Read the model definition and answer for the solid it produces. Units are mm, in the model's axes. A direction names the side the tool comes from. Give positions to 0.01 mm unless a question says otherwise; leave off trailing zeros. Write each loop counter-clockwise with the first axis right and the second up, starting at its lowest first coordinate (ties: lowest second). Pieces come first, ordered by that corner, then holes. Notation, with made-up numbers: M 42,26 L 49,26 A36 cw 49,62 Z; hole C 57.25,-10.75 d8. An arc over 180 degrees is marked long. Use a Markdown table: item, result. Add a question column.
Item 1: A cutting plane is placed at B-B on y = 1. Determine the outline of the cut face in (x, z), then the cut area to 3 significant figures.
Item 2: A cutting plane is placed at D-D on z = 2.25. Determine the outline of the cut face in (x, y).
Item 3: A cutting plane is placed at A-A on z = 4.25. Determine the outline of the cut face in (x, y), then the cut area to 3 significant figures.
Item 4: Consider probe 1 along X at (y, z) = (4.5, -2.25); probe 2 along X at (y, z) = (5.25, 3.5); probe 3 along X at (y, z) = (8.5, -5.25). Determine where each line is inside the solid, lowest interval first. Write a range as [from, to].
Item 5: A cutting plane is placed at C-C on y = 7.5. Determine the outline of the cut face in (x, z), then the cut area to 3 significant figures.
Item 6: For faces 1 (the flat face through (4, 15, 0)), 2 (the flat face through (-8, 8, -3.027)), determine the directions among +Z, -Z, +X, -X, +Y, -Y from which every point of the face is accessible in a straight line to the end or side of a thin tool.
Item 7: The mould has two halves that part along X. Classify faces 3 (the flat face through (17.5, 7, 0)), 4 (the cylindrical face through (-15.273, 7.906, 5.479)), 5 (the flat face through (-8, 6, 3.027)), 6 (the cylindrical face through (-11.704, 8.852, 5.548)): pulls with the +X half, pulls with the -X half, needs draft (parallel to the pull), parting line crosses it, or undercut.
Item 8: Given P1, Ø1.8, axis at y = 5, z = 1.5, coming from the -X side; P2, Ø8, axis at y = 6, z = 5, coming from the -X side, each flat-ended and moving along its own axis, determine where each tip first touches the part or whether it passes through.
from build123d import *

# Parameters (mm, degrees)
SKETCH_1_W          = 35
SKETCH_1_H          = 16
EXTRUDE_1_DEPTH     = 15
SKETCH_2_W          = 27.377038818
SKETCH_2_H          = 6.053774878
CUT_EXTRUDE_2_DEPTH = 25.397745798
SKETCH_3_R          = 2
CUT_EXTRUDE_3_DEPTH = 29.057975693
CHAMFER_1_SIZE      = 8.342275148
CHAMFER_1_SIZE_2    = 7
FILLET_1_R          = 5


with BuildPart() as part:
    # Эскиз1 → Вытянуть1 (new body)
    with BuildSketch(Plane(origin=(0, 0, 0), x_dir=(1, 0, 0), z_dir=(0, 1, 0))):
        Rectangle(SKETCH_1_W, SKETCH_1_H)
    extrude(amount=EXTRUDE_1_DEPTH)

    # Эскиз2 → Вытянуть2 (cut, through all)
    with BuildSketch(Plane(origin=(0, 15, 0), x_dir=(1, 0, 0), z_dir=(0, 1, 0))):
        with Locations((-17.5, 0)):
            Rectangle(SKETCH_2_W, SKETCH_2_H)
    extrude(amount=-CUT_EXTRUDE_2_DEPTH, mode=Mode.SUBTRACT)

    # Эскиз3 → Вытянуть3 (cut, through all)
    with BuildSketch(Plane.XY.offset(8)):
        with Locations((-10.229823295, 7.5)):
            Circle(SKETCH_3_R)
    extrude(amount=-CUT_EXTRUDE_3_DEPTH, mode=Mode.SUBTRACT)

    # Фаска1
    # the kernel refuses this chamfer: 8.342275148, 7 mm, written as the material it takes off along each edge
    with BuildSketch(Plane(origin=(-17.5, 0, 18.474543444), x_dir=(-0.024939322090234327, 0.9996889667359942, 0), z_dir=(0, 0, -1)), Plane(origin=(-17.5, 15, 29.501430883), x_dir=(0.9996889667359942, 0.024939322090234327, 0), z_dir=(0, 0, -1))) as chamfer_1_piece_1:
        Polygon((CHAMFER_1_SIZE * 0.999688966755, CHAMFER_1_SIZE * 0.0249393220907), (-CHAMFER_1_SIZE_2 * 0.0249393220902, CHAMFER_1_SIZE_2 * 0.999688966736), (0, 0), align=None)
    extrude(amount=47.975974327, mode=Mode.SUBTRACT)
    with BuildSketch(Plane(origin=(-17.5, 0, 29.501430883), x_dir=(0.9993728857116146, -0.03540953691366304, 0), z_dir=(0, 0, -1)), Plane(origin=(-17.5, 15, 18.474543444), x_dir=(-0.035409536913663095, -0.9993728857116146, 0), z_dir=(0, 0, -1))) as chamfer_1_piece_2:
        Polygon((CHAMFER_1_SIZE_2 * 0.999372885712, -CHAMFER_1_SIZE_2 * 0.0354095369137), (-CHAMFER_1_SIZE * 0.0354095369143, -CHAMFER_1_SIZE * 0.999372885731), (0, 0), align=None)
    extrude(amount=47.975974327, mode=Mode.SUBTRACT)

    # Скругление1
    fillet_1_edges = [part.edges().sort_by_distance(p)[0] for p in [
        (-17.33146239, 8.141419846, 5.513443719),
    ]]
    fillet(fillet_1_edges, radius=FILLET_1_R)


solid = part.part
Filled in:
| question | item | result |
|---|---|---|
| 1 | outline | M -11.34,-8 L 17.5,-8 L 17.5,8 L -11.34,8 L -11.34,3.03 L -3.81,3.03 L -3.81,-3.03 L -11.34,-3.03 Z |
| 1 | area | 416 mm² |
| 2 | outline | M -3.81,0 L 17.5,0 L 17.5,15 L -3.81,15 Z |
| 3 | outline | M -14.12,4.31 L -10.5,0 L 17.5,0 L 17.5,15 L -9.16,15 L -13.5,11.36 A5 ccw Z; hole C -10.23,7.5 d4 |
| 3 | area | 449 mm² |
| 4 | probe 1 | [-3.81, 17.5] |
| 4 | probe 2 | [-14.74, 17.5] |
| 4 | probe 3 | [-16.9, -11.96], [-8.5, 17.5] |
| 5 | outline | M -16.79,-8 L -12.23,-8 L -12.23,-3.03 L -16.79,-3.03 Z; M -15.29,3.03 L -12.23,3.03 L -12.23,8 L -15.29,8 Z; M -8.23,-8 L 17.5,-8 L 17.5,8 L -8.23,8 L -8.23,3.03 L -3.81,3.03 L -3.81,-3.03 L -8.23,-3.03 Z |
| 5 | area | 423 mm² |
| 6 | face 1 | +Z, -Z, +X, -X, +Y |
| 6 | face 2 | -X, +Y, -Y |
| 7 | face 3 | pulls with the +X half |
| 7 | face 4 | pulls with the -X half |
| 7 | face 5 | needs draft |
| 7 | face 6 | undercut |
| 8 | P1 | x = -3.81 |
| 8 | P2 | x = -15.29 |
